Part model, mm, in its own coordinate system. A direction names the side the tool comes from. Give positions to 0.01 mm unless a question says otherwise; leave off trailing zeros. Write each loop counter-clockwise with the first axis right and the second up, starting at its lowest first coordinate (ties: lowest second). Pieces come first, ordered by that corner, then holes. Notation, with made-up numbers: M -15,85 L 40,85 A12 ccw 40,107 Z; hole C 41,6 d11. An arc over 180 degrees is marked long. Answer as CSV lines item,"result". Start each with the question number.
1) Tool access for faces 1 (the flat face through (0, 0, 0)), 2 (the flat face through (6.5, -3, 4)), 3 (the cylindrical face through (-26.442, -4.124, 2.465)): list every direction of +Z, -Z, +X, -X, +Y, -Y with a clear straight run to the whole face (end or side of a thin tool).
2) Slice it at D-D, the plane y = -0.75. Give the cut face in (x, z) (3 decimals).
3) Slice it at B-B, the plane y = -7.5. Give the cut face in (x, z).
4) Slice it at A-A, the plane x = 2.5. Give the cut face in (y, z), plus the area to 3 significant figures.
5) Mould opens along Y. For faces 4 (the flat face through (-31.5, 0, 2)), 5 (the cylindrical face through (26.442, 11.124, 2.465)), 6 (the flat face through (0, -12.5, 2)), 7 (the flat face through (-7, -4.25, 4)) say: pulls with the +Y half, pulls with the -Y half, needs draft (parallel to the pull), parting line crosses it, or undercut.
6) Wall check: line 1 along X through (y, z) = (2.25, 3.2) (3 decimals); line 2 along X through (y, z) = (7, 3.4) (3 decimals); line 3 along X through (y, z) = (0.25, 3.25) (3 decimals). Give the ranges that are in metal, low to high. Write a range as from..to.
7) Slice it at C-C, the plane x = -13. Give the cut face in (y, z), plus the area to 3 significant figures.
8) Pin check, flat tip, straight feed: pin 1 Ø1.5 at (x, y) = (-3, -2) entering from +Z. Stop position of the tip, or through.
Autodesk Fusion 360 part; units mm, degrees
sketch "Sketch1" plane through (0, 0, 0) normal (0, 0, 1) x (1, 0, 0)
  line L0 (31.5, -12.5) -> (-31.5, -12.5)
  line L1 (-31.5, -12.5) -> (-31.5, 12.5)
  line L2 (-31.5, 12.5) -> (31.5, 12.5)
  line L3 (31.5, 12.5) -> (31.5, -12.5)
  line L4 (31.5, -12.5) -> (-31.5, 12.5) construction
  line L5 (-31.5, -12.5) -> (31.5, 12.5) construction
  circle A0 centre (-16.5, -7.5) radius 1.5
  circle A1 centre (2.5, -7.5) radius 1.5
  line L6 (-29.125, 8.5) -> (-29.125, -1.5)
  arc A2 (-29.125, -1.5) -> (-23.875, -1.5) centre (-26.5, -1.5) ccw
  line L7 (-23.875, -1.5) -> (-23.875, 8.5)
  arc A3 (-23.875, 8.5) -> (-29.125, 8.5) centre (-26.5, 8.5) ccw
  line L8 (-26.5, 8.5) -> (-26.5, -1.5) construction
  line L9 (29.125, -1.5) -> (29.125, 8.5)
  arc A4 (29.125, 8.5) -> (23.875, 8.5) centre (26.5, 8.5) ccw
  line L10 (23.875, 8.5) -> (23.875, -1.5)
  arc A5 (23.875, -1.5) -> (29.125, -1.5) centre (26.5, -1.5) ccw
  line L11 (26.5, -1.5) -> (26.5, 8.5) construction
  line L12 (-14.25, 0.75) -> (0.75, 0.75)
  line L13 (0.75, 0.75) -> (0.75, -4.25)
  line L14 (0.75, -4.25) -> (-14.25, -4.25)
  line L15 (-14.25, -4.25) -> (-14.25, 0.75)
  line L16 (-14.25, -1.75) -> (0.75, -1.75) construction
  line L17 (6.5, 2.5) -> (11.5, 2.5)
  line L18 (11.5, 2.5) -> (11.5, -8.5)
  line L19 (11.5, -8.5) -> (6.5, -8.5)
  line L20 (6.5, -8.5) -> (6.5, 2.5)
  line L21 (9, 2.5) -> (9, -8.5) construction
  line L22 (-6.75, 0.75) -> (-6.75, -4.25) construction
  dimension "d1" = 63
  dimension "d2" = 25
  dimension "d3" = 3
  dimension "d4" = 3
  dimension "d5" = 19
  dimension "d6" = 5
  dimension "d7" = 5
  dimension "d8" = 15
  dimension "d9" = 5.25
  dimension "d10" = 5.25
  dimension "d11" = 5
  dimension "d12" = 5
  dimension "d15" = 4
  dimension "d16" = 4
  dimension "d17" = 10
  dimension "d18" = 10
  dimension "d19" = 5
  dimension "d20" = 5.75
  dimension "d21" = 5
  dimension "d22" = 15
  dimension "d23" = 2.25
  dimension "d24" = 11
  dimension "d25" = 6.5
  dimension "d26" = 1
extrude "Extrude1" add sketch "Sketch1" along normal blind 5 contours L0 L1 L2 L3 | L12 L13 L14 L15 | L17 L18 L19 L20
extrude "Extrude2" cut sketch "Sketch1" against normal blind 2.5 from surface at 5 contours L12 L13 L14 L15 | L17 L18 L19 L20
chamfer "Chamfer1" distance 0.4 angle 45 8 edges at (-6.75, 0.75, 5) (-14.25, -1.75, 5) (-6.75, -4.25, 5) (0.75, -1.75, 5) (9, 2.5, 5) (6.5, -3, 5) (11.5, -3, 5) (9, -8.5, 5)
equation "d7 = d6"
equation "d10 = d9"
equation "d12 = d11"
equation "d16 = d15"
equation "d18 = d17"
Found:
1,face 1,"-Z, +X, -X, +Y, -Y"
1,face 2,"+Z"
1,face 3,"+Z, -Z"
2,outline,"M -31.5,0 L -29.125,0 L -29.125,5 L -31.5,5 Z; M -23.875,0 L 23.875,0 L 23.875,5 L 11.9,5 L 11.5,4.6 L 11.5,2.5 L 6.5,2.5 L 6.5,4.6 L 6.1,5 L 1.15,5 L 0.75,4.6 L 0.75,2.5 L -14.25,2.5 L -14.25,4.6 L -14.65,5 L -23.875,5 Z; M 29.125,0 L 31.5,0 L 31.5,5 L 29.125,5 Z"
3,outline,"M -31.5,0 L -18,0 L -18,5 L -31.5,5 Z; M -15,0 L 1,0 L 1,5 L -15,5 Z; M 4,0 L 31.5,0 L 31.5,5 L 11.9,5 L 11.5,4.6 L 11.5,2.5 L 6.5,2.5 L 6.5,4.6 L 6.1,5 L 4,5 Z"
4,outline,"M -12.5,0 L -9,0 L -9,5 L -12.5,5 Z; M -6,0 L 12.5,0 L 12.5,5 L -6,5 Z"
4,area,"110 mm²"
5,face 4,"needs draft"
5,face 5,"undercut"
5,face 6,"pulls with the -Y half"
5,face 7,"undercut"
6,line 1,"-31.5..-29.125, -23.875..6.5, 11.5..23.875, 29.125..31.5"
6,line 2,"-31.5..-29.125, -23.875..23.875, 29.125..31.5"
6,line 3,"-31.5..-29.125, -23.875..-14.25, 0.75..6.5, 11.5..23.875, 29.125..31.5"
7,outline,"M -12.5,0 L 12.5,0 L 12.5,5 L 1.15,5 L 0.75,4.6 L 0.75,2.5 L -4.25,2.5 L -4.25,4.6 L -4.65,5 L -12.5,5 Z"
7,area,"112 mm²"
8,pin 1,"z = 2.5"
